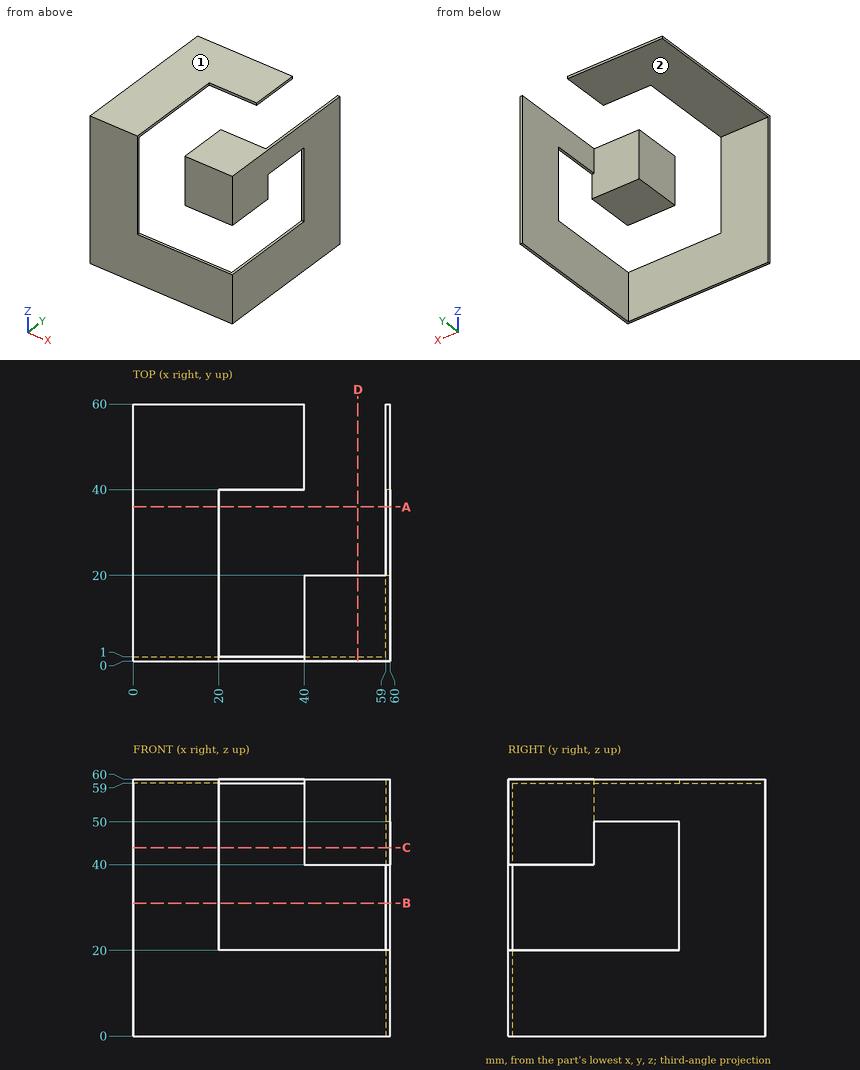
For this review, use the dimensioned drawing (mm, ordinates from the lowest corner) and the shaded views. A direction names the side the tool comes from. Round coordinates to 2 decimals unless told otherwise and drop trailing zeros. Loops run counter-clockwise (first coordinate to the right, second up) from the corner with the lowest first, then second, coordinate; pieces in that order, holes last. Notation, with made-up numbers: M 85.5,79 L 129.5,79 A26 cw 129.5,94 Z; hole C -37,20.25 d11. An arc over 180 degrees is marked long. Answer as a JSON object with one key per item and string values.
(1) To check wall thickness, follow line 1 along Y through (x, z) = (12.5, 39.5); line 2 along X through (y, z) = (44, 23). State the ranges of each line that lie inside material, in increasing order.
Resolved:
{"line 1": "0 to 1", "line 2": "59 to 60"}
(2) Tool access review of the marked faces 1 and 2: name each direction out of +Z, -Z, +X, -X, +Y, -Y from which nothing blocks a thin tool from reaching the whole face with its end or side.
Resolved:
{"face 1": "+Z, +X, -X, +Y, -Y", "face 2": "-Z, -X, +Y"}
(3) Take a section at C-C on z = 44. Give the boundary of the cut face in (x, y).
Resolved:
{"outline": "M 0,0 L 20,0 L 20,1 L 0,1 Z; M 40,0 L 60,0 L 60,20 L 40,20 Z; M 59,40 L 60,40 L 60,60 L 59,60 Z"}
(4) Clearance check with flat-ended pins moving along their axes: P1, Ø20, axis at x = 13, y = 26.5, coming from the -Z side; P2, Ø12, axis at x = 36, y = 33.5, coming from the -Z side; P3, Ø10, axis at x = 46.5, z = 49.5, coming from the +Y side; P4, Ø4, axis at y = 32.5, z = 8.5, coming from the -X side. State where each tip first meets the part, or that it passes through.
Resolved:
{"P1": "z = 59", "P2": "through", "P3": "y = 20", "P4": "x = 59"}
(5) Take a section at B-B on z = 31. Give the boundary of the cut face in (x, y), and give its area (3 significant figures).
Resolved:
{"outline": "M 0,0 L 20,0 L 20,1 L 0,1 Z; M 59,40 L 60,40 L 60,60 L 59,60 Z", "area": "40.0 mm²"}
(6) Take a section at A-A on y = 36. Give the boundary of the cut face in (x, z).
Resolved:
{"outline": "M 0,59 L 20,59 L 20,60 L 0,60 Z; M 59,0 L 60,0 L 60,20 L 59,20 Z; M 59,50 L 60,50 L 60,60 L 59,60 Z"}
(7) Take a section at D-D on x = 52.5. Give the boundary of the cut face in (y, z).
Resolved:
{"outline": "M 0,0 L 1,0 L 1,20 L 0,20 Z; M 0,40 L 20,40 L 20,60 L 0,60 Z"}
